Could you check a few things on this model? Use its own coordinates, in mm. A direction names the side the tool comes from. Give positions to 0.01 mm unless a question says otherwise; leave off trailing zeros. Order: outer loops, then holes, each group sorted by start corner. A loop starts at its lowest first (then second) coordinate and runs counter-clockwise, first axis right, second up.
(1) Imagine slicing it at D-D, the plane z = -29. Write out the boundary of the cut face in (x, y).
(2) If I drill on probe 1 along X at (y, z) = (-53.5, -4); probe 2 along Y at (x, z) = (26.5, -22.5), over which ranges is the centre line in solid material (lowest first)?
(3) Imagine slicing it at A-A, the plane y = 0. Write out the boundary of the cut face in (x, z).
(4) Imagine slicing it at C-C, the plane x = 14. Write out the boundary of the cut face in (y, z).
(5) Imagine slicing it at B-B, the plane z = -71. Write out the boundary of the cut face in (x, y), then the cut area to 3 significant figures.
(6) On a 3-axis mill with a long thin cutter (end or side, diameter ignored), from which of +Z, -Z, +X, -X, +Y, -Y can I reach the whole of each face in a straight line? I mean faces 5 (the flat face through (-44, -1, -48)), 6 (the flat face through (-45, 6, -80)). Say none if no direction works.
(7) If we mould it in two halves opening along Y, with no side actions, what happens to faces 1 (the flat face through (-1, 75, -39)), 2 (the flat face through (-50, -1, -48)), 3 (the cylindrical face through (46.96, -0.88, -39.99)), 4 (the flat face through (44, -1, -48))? For each: released by +Y, released by -Y, zero draft, split by the parting line, or undercut.
from build123d import *

# Parameters (mm, degrees)
SKETCH1_W               = 100
SKETCH1_H               = 150
SKETCH1_W_2             = 88
SKETCH1_H_2             = 138
BOSS_EXTRUDE1_DEPTH     = 80
SKETCH2_R               = 40
CUT_EXTRUDE1_DEPTH      = 51
CUT_EXTRUDE1_DEPTH_BACK = 51


with BuildPart() as part:
    # Sketch1 → Boss-Extrude1 (new body)
    with BuildSketch(Plane.XY):
        Rectangle(SKETCH1_W, SKETCH1_H)
        Rectangle(SKETCH1_W_2, SKETCH1_H_2, mode=Mode.SUBTRACT)
    extrude(amount=-BOSS_EXTRUDE1_DEPTH)

    # Sketch2 → Cut-Extrude1 (cut, two sides)
    with BuildSketch(Plane(origin=(0, 0, 0), x_dir=(0, 0, -1), z_dir=(1, 0, 0))) as cut_extrude1_sk:
        Circle(SKETCH2_R)
    extrude(amount=CUT_EXTRUDE1_DEPTH, mode=Mode.SUBTRACT)
    extrude(cut_extrude1_sk.sketch, amount=-CUT_EXTRUDE1_DEPTH_BACK, mode=Mode.SUBTRACT)


solid = part.part
Answer block:
1. outline: (-50, -75) - (50, -75) - (50, -27.55) - (44, -27.55) - (44, -69) - (-44, -69) - (-44, -27.55) - (-50, -27.55) - close; (-50, 27.55) - (-44, 27.55) - (-44, 69) - (44, 69) - (44, 27.55) - (50, 27.55) - (50, 75) - (-50, 75) - close
2. probe 1: x = -50 to -44, 44 to 50
2. probe 2: y = -75 to -69, 69 to 75
3. outline: (-50, -80) - (-44, -80) - (-44, -40) - (-50, -40) - close; (44, -80) - (50, -80) - (50, -40) - (44, -40) - close
4. outline: (-75, -80) - (-69, -80) - (-69, 0) - (-75, 0) - close; (69, -80) - (75, -80) - (75, 0) - (69, 0) - close
5. outline: (-50, -75) - (50, -75) - (50, 75) - (-50, 75) - close; hole (-44, -69) - (44, -69) - (44, 69) - (-44, 69) - close
5. area: 2,860 mm2
6. face 5: +Z, -Z
6. face 6: -Z, +X, -X, +Y, -Y
7. face 1: released by +Y
7. face 2: zero draft
7. face 3: undercut
7. face 4: undercut
